Verification items for the finished model (mm, model axes). Give positions to 0.01 mm unless a question says otherwise; leave off trailing zeros. Use a Markdown table: item, result.
from build123d import *

# Parameters (mm, degrees)
F2_DEPTH = 2.5
F1_R     = 2.5
F3_DEPTH = 3
F4_DEPTH = 3


with BuildPart() as f2:
    # F0 (on Front) → F2 (new body)
    with BuildSketch(Plane.XZ):
        with BuildLine():
            add(Edge.make_bspline(
                [(-96.9805282175, -0.8100506688), (-84.7869920978, 5.1468541776), (-43.2313518226, 10.3846705605), (26.8477938201, 4.0208678603), (73.1462007926, -1.0427900778)],
                knots=[0, 0, 0, 0, 0.374886421, 0.9004696716, 0.9004696716, 0.9004696716, 0.9004696716], degree=3))
            add(Edge.make_bspline(
                [(-97.5447368223, -7.1186651935), (-99.939251346, -6.5508492693), (-102.885147974, -5.168950634), (-100.0067471137, -2.3789404522), (-96.9805282175, -0.8100506688)],
                knots=[0.0564585679, 0.0564585679, 0.0564585679, 0.0564585679, 0.4847104148, 1, 1, 1, 1], degree=3))
            add(Edge.make_bspline(
                [(-96.5428845142, -7.3406707446), (-96.8949965543, -7.2673488468), (-97.22905608, -7.1935231869), (-97.5447368223, -7.1186651935)],
                knots=[0, 0, 0, 0, 0.0564585679, 0.0564585679, 0.0564585679, 0.0564585679], degree=3))
            add(Edge.make_bspline(
                [(-96.5428845142, -7.3406707446), (-80.7020161693, -9.4302402111), (-44.2471235075, -11.1181020976), (27.9226364637, -4.7767282079), (62.4434148738, -4.5021877215), (71.7967184236, -4.4503783305)],
                knots=[0, 0, 0, 0, 0.2987594418, 0.6837410955, 0.8381168975, 0.8381168975, 0.8381168975, 0.8381168975], degree=3))
            Line((71.7967184236, -4.4503783305), (72.2670713195, -3.2626866351))
            add(Edge.make_bspline(
                [(-97.3825784566, -6.0471531808), (-82.3468325761, -8.841713568), (-44.2551066449, -8.6286827794), (32.5707299039, -3.8332069517), (63.1103828262, -3.2710139005), (72.2670713195, -3.2626866351)],
                knots=[0, 0, 0, 0, 0.3131273629, 0.7122131732, 0.9019797674, 0.9019797674, 0.9019797674, 0.9019797674], degree=3))
            add(Edge.make_bspline(
                [(-97.3825784566, -6.0471531808), (-98.6588937786, -5.8946130057), (-100.1661659123, -5.1778479876), (-99.9138553768, -4.2244412327), (-99.8196757147, -4.047003109)],
                knots=[0, 0, 0, 0, 0.4440177242, 0.5425000514, 0.5425000514, 0.5425000514, 0.5425000514], degree=3))
            add(Edge.make_bspline(
                [(-99.8196757147, -4.047003109), (-99.3821638101, -3.2227137691), (-97.9006497107, -2.3042858417), (-96.3385477662, -1.6362179573)],
                knots=[0.5425000514, 0.5425000514, 0.5425000514, 0.5425000514, 1, 1, 1, 1], degree=3))
            add(Edge.make_bspline(
                [(-96.3385477662, -1.6362179573), (-85.7442874691, 3.2900694446), (-41.4192830911, 9.6956733525), (28.5693195485, 2.5855104747), (72.7689680214, -1.9953434339)],
                knots=[0, 0, 0, 0, 0.384923117, 0.9441251659, 0.9441251659, 0.9441251659, 0.9441251659], degree=3))
            Line((72.7689680214, -1.9953434339), (73.1462007926, -1.0427900778))
        make_face()
        with BuildLine():
            add(Edge.make_bspline(
                [(-96.5428845142, -7.3406707446), (-96.8949965543, -7.2673488468), (-97.22905608, -7.1935231869), (-97.5447368223, -7.1186651935)],
                knots=[0, 0, 0, 0, 0.0564585679, 0.0564585679, 0.0564585679, 0.0564585679], degree=3))
            ThreePointArc((-97.5447368223, -7.1186651935), (-97.052492706, -7.2688477084), (-96.5428845142, -7.3406707446))
        make_face()
        with BuildLine():
            Line((72.2670713195, -3.2626866351), (72.7689680214, -1.9953434339))
            add(Edge.make_bspline(
                [(-96.3385477662, -1.6362179573), (-85.7442874691, 3.2900694446), (-41.4192830911, 9.6956733525), (28.5693195485, 2.5855104747), (72.7689680214, -1.9953434339)],
                knots=[0, 0, 0, 0, 0.384923117, 0.9441251659, 0.9441251659, 0.9441251659, 0.9441251659], degree=3))
            add(Edge.make_bspline(
                [(-99.8196757147, -4.047003109), (-99.3821638101, -3.2227137691), (-97.9006497107, -2.3042858417), (-96.3385477662, -1.6362179573)],
                knots=[0.5425000514, 0.5425000514, 0.5425000514, 0.5425000514, 1, 1, 1, 1], degree=3))
            add(Edge.make_bspline(
                [(-97.3825784566, -6.0471531808), (-98.6588937786, -5.8946130057), (-100.1661659123, -5.1778479876), (-99.9138553768, -4.2244412327), (-99.8196757147, -4.047003109)],
                knots=[0, 0, 0, 0, 0.4440177242, 0.5425000514, 0.5425000514, 0.5425000514, 0.5425000514], degree=3))
            add(Edge.make_bspline(
                [(-97.3825784566, -6.0471531808), (-82.3468325761, -8.841713568), (-44.2551066449, -8.6286827794), (32.5707299039, -3.8332069517), (63.1103828262, -3.2710139005), (72.2670713195, -3.2626866351)],
                knots=[0, 0, 0, 0, 0.3131273629, 0.7122131732, 0.9019797674, 0.9019797674, 0.9019797674, 0.9019797674], degree=3))
        make_face()
    extrude(amount=F2_DEPTH)


with BuildPart() as f2b:
    # F1 (on Front) → F2, piece 2 (new body)
    with BuildSketch(Plane.XZ):
        with BuildLine():
            ThreePointArc((-45.542362095, -1.3708024857), (-51.4789804014, 2.1291274472), (-51.6671168627, -4.7598166753))
            Line((-51.6671168627, -4.7598166753), (-47.385046135, -4.7391830831))
            ThreePointArc((-47.385046135, -4.7391830831), (-46.0331411102, -3.2905337378), (-45.542362095, -1.3708024857))
        make_face()
        with BuildLine():
            Line((-47.385046135, -4.7391830831), (-51.6671168627, -4.7598166753))
            ThreePointArc((-51.6671168627, -4.7598166753), (-49.523087913, -5.3707560487), (-47.385046135, -4.7391830831))
        make_face()
    extrude(amount=F2_DEPTH)


with BuildPart() as f2c:
    # F1 (on Front) → F2, piece 3 (new body)
    with BuildSketch(Plane.XZ):
        with Locations((33.7789729238, -1.0305350879)):
            Circle(F1_R)
    extrude(amount=F2_DEPTH)


with BuildPart() as f3_tool:
    # F3 (cut): a face of the model
    f3_faces = [f2b.part.faces().sort_by_distance(p)[0] for p in [
        (-49.542362095, -2.5, -1.3708024857),
    ]]
    extrude(f3_faces, amount=-F3_DEPTH)


with BuildPart() as f2_1:
    add(f2.part)

    # F3: cut by f3_tool
    add(f3_tool.part, mode=Mode.SUBTRACT)


with BuildPart() as f2b_1:
    add(f2b.part)

    # F3: cut by f3_tool
    add(f3_tool.part, mode=Mode.SUBTRACT)


with BuildPart() as f4_tool:
    # F4 (cut): a face of the model
    f4_faces = [f2c.part.faces().sort_by_distance(p)[0] for p in [
        (33.7789729238, -2.5, -1.0305350879),
    ]]
    extrude(f4_faces, amount=-F4_DEPTH)


with BuildPart() as f2_2:
    add(f2_1.part)

    # F4: cut by f4_tool
    add(f4_tool.part, mode=Mode.SUBTRACT)


with BuildPart() as f2c_1:
    add(f2c.part)

    # F4: cut by f4_tool
    add(f4_tool.part, mode=Mode.SUBTRACT)


solid = f2_2.part
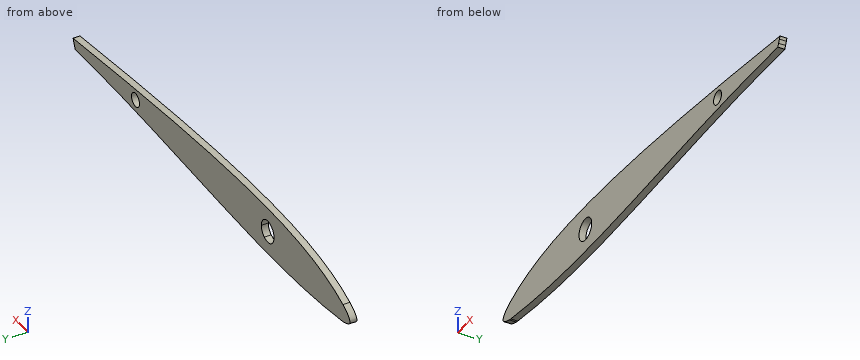
(1) Cross-section at A-A on y = -1.65. State how many separate pieces and enclosed holes the cut face has, then the cut area to 3 significant figures.
Results below:
| item | result |
|---|---|
| separate pieces | 1 |
| enclosed holes | 2 |
| area | 1,980 mm^2 |
(2) Material ranges on line 1 (X direction, y = -0.6, z = -2); line 2 (X direction, y = -0.8, z = -3); line 3 (Z direction, x = -52, y = -0.7), recorded low to high.
Results below:
| item | result |
|---|---|
| line 1 | -99.01 to -53.49, -45.59 to 31.47, 36.08 to 72.77 |
| line 2 | -100.31 to -53.2, -45.89 to 32.24, 35.32 to 72.37 |
| line 3 | -9.75 to -4.53, 1.79 to 7.38 |
(3) Gauge pin test, flat ends, axial feed: P1, Ø1, axis at x = -68.5, y = -1, coming from the -Z side; P2, Ø8, axis at x = 33.78, z = -1.03, coming from the +Y side; P3, Ø1.5, axis at x = -31.5, y = -0.5, coming from the -Z side. Record the tip position at first contact, or that the pin passes through.
Results below:
| item | result |
|---|---|
| P1 | z = -9.62 |
| P2 | y = 0 |
| P3 | z = -9.12 |
